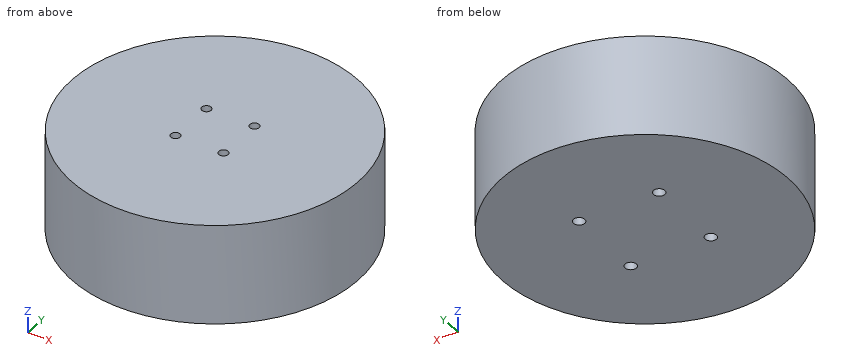
```python
from build123d import *

# Parameters (mm, degrees)
SKETCH1_R                          = 31.5
BOSS_EXTRUDE1_DEPTH                = 22
TAP_DRILL_FOR_M2_5X0_45_TAP1_D     = 2.05
TAP_DRILL_FOR_M2_5X0_45_TAP1_DEPTH = 5.5
TAP_DRILL_FOR_M2_5X0_45_TAP1_TIP   = 0.615882135
TAP_DRILL_FOR_M3X0_5_TAP1_D        = 2.5
TAP_DRILL_FOR_M3X0_5_TAP1_DEPTH    = 5.5
TAP_DRILL_FOR_M3X0_5_TAP1_TIP      = 0.751075774


with BuildPart() as part:
    # Sketch1 → Boss-Extrude1 (new body)
    with BuildSketch(Plane.XY):
        Circle(SKETCH1_R)
    extrude(amount=BOSS_EXTRUDE1_DEPTH)

    # Tap Drill for M2.5x0.45 Tap1
    with Locations(Plane.XY.offset(22)):
        with Locations((-5.303300859, 5.303300859), (5.303300859, -5.303300859), (5.303300859, 5.303300859), (-5.303300859, -5.303300859)):
            Hole(TAP_DRILL_FOR_M2_5X0_45_TAP1_D / 2, depth=TAP_DRILL_FOR_M2_5X0_45_TAP1_DEPTH)
            with Locations((0, 0, -(TAP_DRILL_FOR_M2_5X0_45_TAP1_DEPTH + TAP_DRILL_FOR_M2_5X0_45_TAP1_TIP / 2))):  # 118° drill point
                Cone(0, TAP_DRILL_FOR_M2_5X0_45_TAP1_D / 2, TAP_DRILL_FOR_M2_5X0_45_TAP1_TIP, mode=Mode.SUBTRACT)

    # Tap Drill for M3x0.5 Tap1
    with Locations(Plane(origin=(0, 0, 0), x_dir=(-1, 0, 0), z_dir=(0, 0, -1))):
        with Locations((8.838834765, 8.838834765), (8.838834765, -8.838834765), (-8.838834765, 8.838834765), (-8.838834765, -8.838834765)):
            Hole(TAP_DRILL_FOR_M3X0_5_TAP1_D / 2, depth=TAP_DRILL_FOR_M3X0_5_TAP1_DEPTH)
            with Locations((0, 0, -(TAP_DRILL_FOR_M3X0_5_TAP1_DEPTH + TAP_DRILL_FOR_M3X0_5_TAP1_TIP / 2))):  # 118° drill point
                Cone(0, TAP_DRILL_FOR_M3X0_5_TAP1_D / 2, TAP_DRILL_FOR_M3X0_5_TAP1_TIP, mode=Mode.SUBTRACT)


solid = part.part
```
Here's how the part is built. I have some questions about the finished solid (model axes, mm). Round coordinates to 2 decimals unless told otherwise and drop trailing zeros. Order: outer loops, then holes, each group sorted by start corner. A loop starts at its lowest first (then second) coordinate and runs counter-clockwise, first axis right, second up. Notation, with made-up numbers: (70.5, 42.5) -> (125.5, 42.5) arc R20 cw to (125.5, 55.5) -> close; hole circle Ø5 at (45, 55.5). An arc over 180 degrees is marked (long way). Use a Markdown table: item, result. Add a question column.
(1) Suppose I cut it at B-B, the plane y = 23.5. Please give me the cut outline in (x, z).
(2) Suppose I cut it at D-D, the plane x = -24. Please give me the cut outline in (y, z), and give its area (3 significant figures).
(3) For pin 1 Ø1.6 at (x, y) = (5.3, 5.3) entering from +Z; pin 2 Ø12 at (x, z) = (-16, 10) entering from -Y; pin 3 Ø5 at (y, z) = (10, 7.5) entering from +X, each with a flat end and sliding along its axis, tell me the tip position at first contact or that it passes through.
(4) I need wall thicknesses on line 1 along X through (y, z) = (9, 3.75); line 2 along X through (y, z) = (0.5, 3); line 3 along X through (y, z) = (-15.5, 4.75). Which ranges of each line are inside material? Lowest first, please.
(5) Suppose I cut it at A-A, the plane z = 7. Please give me the cut outline in (x, y).
(6) Suppose I cut it at C-C, the plane z = 20.75. Please give me the cut outline in (x, y) (3 decimals).
Verdict:
| question | item | result |
|---|---|---|
| 1 | outline | (-20.98, 0) -> (20.98, 0) -> (20.98, 22) -> (-20.98, 22) -> close |
| 2 | outline | (-20.4, 0) -> (20.4, 0) -> (20.4, 22) -> (-20.4, 22) -> close |
| 2 | area | 898 mm2 |
| 3 | pin 1 | z = 16.37 |
| 3 | pin 2 | y = -29.87 |
| 3 | pin 3 | x = 30.59 |
| 4 | line 1 | -30.19 to -10.08, -7.6 to 7.6, 10.08 to 30.19 |
| 4 | line 2 | -31.5 to 31.5 |
| 4 | line 3 | -27.42 to 27.42 |
| 5 | outline | circle Ø63 at (0, 0) |
| 6 | outline | circle Ø63 at (0, 0); hole circle Ø2.05 at (-5.303, -5.303); hole circle Ø2.05 at (-5.303, 5.303); hole circle Ø2.05 at (5.303, -5.303); hole circle Ø2.05 at (5.303, 5.303) |
